Verification items for this drawing (mm, ordinates from the low corner). Round coordinates to 2 decimals unless told otherwise and drop trailing zeros. Write each loop counter-clockwise with the first axis right and the second up, starting at its lowest first coordinate (ties: lowest second). Pieces come first, ordered by that corner, then holes. Notation, with made-up numbers: M 64,9 L 112,9 A5 cw 112,17 Z; hole C 23.25,27.5 d10. An arc over 180 degrees is marked long. One line per question, with ' | ' between items. Start each with the question number.
Q1. Gauge pin test, flat end, axial feed: pin 1 (4.5 mm diameter, centred on x = 12.43, z = 10, fed in from +Y). Record the tip position at first contact, or that the pin passes through.
Q2. Cross-section at A-A (z = 10). Record the boundary of the cut face in (x, y).
Q3. Thickness scan on line 1 along X through (y, z) = (4.65, 120); line 2 along Z through (x, y) = (12, 5.6); line 3 along Z through (x, y) = (239, 5.45). Record the ranges inside material, lowest first. Write a range as from..to.
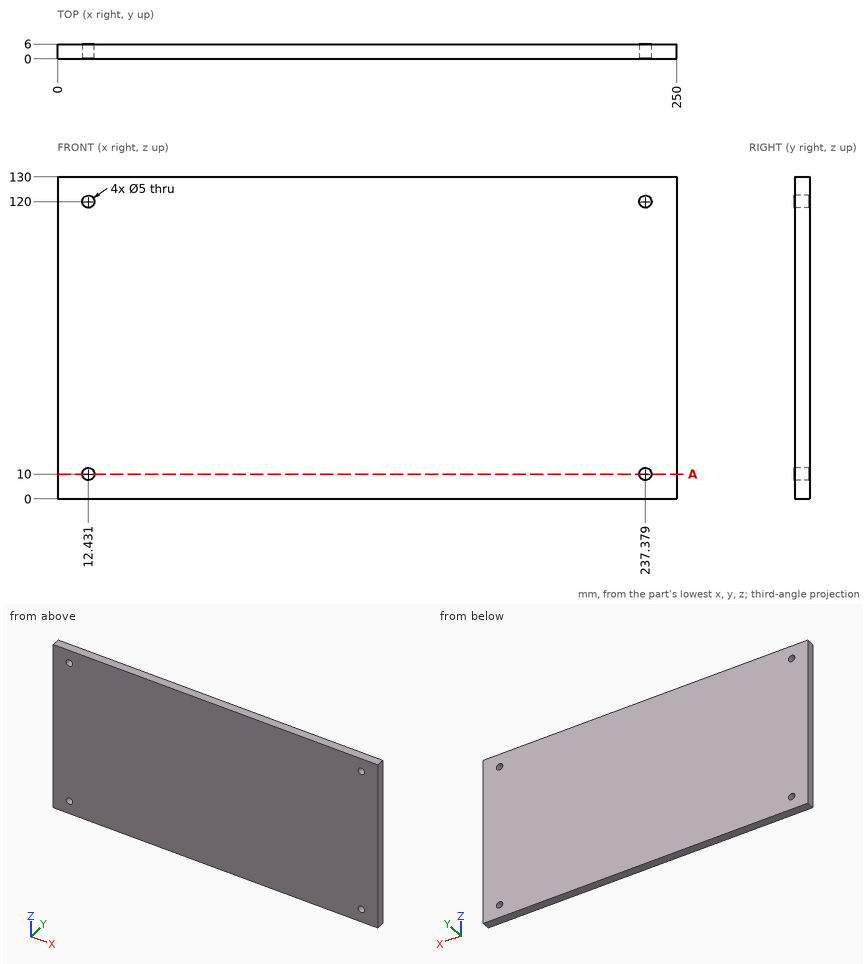
Determined:
1) pin 1: passes through
2) outline: M 0,0 L 9.93,0 L 9.93,6 L 0,6 Z; M 14.93,0 L 234.88,0 L 234.88,6 L 14.93,6 Z; M 239.88,0 L 250,0 L 250,6 L 239.88,6 Z
3) line 1: x = 0..9.93, 14.93..234.88, 239.88..250 | line 2: z = 0..7.54, 12.46..117.54, 122.46..130 | line 3: z = 0..8.1, 11.9..118.1, 121.9..130
